```python
from build123d import *

# Parameters (mm, degrees)
F1_DEPTH  = 15.875
F2_W      = 4.318
F2_H      = 12.7
F3_DEPTH  = 9.175040233
F4_R      = 2.15899
F5_R      = 3.175
F6_DEPTH  = 3.81
F8_DEPTH  = 25.4
F10_DEPTH = 25.4
F11_R     = 3.175


# Not quite as in the source:
# - a fillet or chamfer is up to 0.001 mm smaller than in the source, because OpenCascade refuses the exact size


with BuildPart() as f1:
    # F0 (on Front) → F1 (new body)
    with BuildSketch(Plane.XZ):
        Polygon((9.2045814112, -87.6168819653), (3.0183370735, -43.5994663098), (0, -44.0236659215), (6.1862443377, -88.041081577), align=None)
    extrude(amount=F1_DEPTH)

    # F2 (on face) → F3 (cut, through all)
    with BuildSketch(Plane(origin=(-6.067283434, 0, -0.8527010782), x_dir=(0, -1, 0), z_dir=(-0.9902680687, 0, -0.139173101))):
        with Locations((7.9375, -54.072730631)):
            Rectangle(F2_W, F2_H)
        with Locations((7.9375, -76.297730631)):
            Rectangle(F2_W, F2_H)
    extrude(amount=-F3_DEPTH, mode=Mode.SUBTRACT)

    # F4 (radius 2.159 in the source; OpenCascade refuses exactly that, so slightly less here)
    f4_edges = [f1.edges().sort_by_distance(p)[0] for p in [
        (2.083606, -5.7785, -47.898898),
        (5.176728, -5.7785, -69.907605),
        (5.176728, -10.0965, -69.907605),
        (2.083606, -10.0965, -47.898898),
        (3.851104, -10.0965, -60.475302),
        (6.944226, -10.0965, -82.48401),
        (6.944226, -5.7785, -82.48401),
        (3.851104, -5.7785, -60.475302),
    ]]
    fillet(f4_edges, radius=F4_R)

    # F5 (on Front) → F6 (join)
    with BuildSketch(Plane.XZ):
        Polygon((9.2045814112, -87.6168819653), (3.0183370735, -43.5994663098), (-22.5109767612, -43.5994663098), (-22.5109767612, -25.4), (-73.3109767612, -25.4), (-73.3109767612, -87.6168819653), align=None)
        with Locations((-60.6109767612, -38.1)):
            Circle(F5_R, mode=Mode.SUBTRACT)
    extrude(amount=-F6_DEPTH)

    # F7 (on Front) → F8 (cut)
    with BuildSketch(Plane.XZ):
        Polygon((-73.3109767612, -38.1), (-60.6109767612, -25.4), (-73.3109767612, -25.4), align=None)
    extrude(amount=-F8_DEPTH, mode=Mode.SUBTRACT)

    # F9 (on Front) → F10 (cut)
    with BuildSketch(Plane.XZ):
        Polygon((-74.5969353161, -25.4), (-60.6109767612, -39.3859585549), (-52.9750182062, -31.75), (-22.5109767612, -31.75), (-22.5109767612, -25.4), align=None)
    extrude(amount=-F10_DEPTH, mode=Mode.SUBTRACT)

    # F11
    f11_edges = [f1.edges().sort_by_distance(p)[0] for p in [
        (-67.603956, 1.905, -32.392979),
    ]]
    fillet(f11_edges, radius=F11_R)


solid = f1.part
```
Geometry check sheet. Reference: the model listing, model coordinates, mm. A direction names the side the tool comes from. Give positions to 0.01 mm unless a question says otherwise; leave off trailing zeros. Order: outer loops, then holes, each group sorted by start corner. A loop starts at its lowest first (then second) coordinate and runs counter-clockwise, first axis right, second up. Notation, with made-up numbers: (-8, -18.75) - (24, -18.75) arc R24 ccw to (24, 16.25) - close; hole circle Ø6 at (51, 16). An arc over 180 degrees is marked (long way). Write item = value, one per line. Start each with the question number.
1) Section check B-B (x = -26). Enter the section's corners in (y, z), then the cut area to 3 significant figures.
2) Section check C-C (z = -62.5). Enter the section's corners in (x, y) (3 decimals), then the cut area to 3 significant figures.
3) Draft check along Z on faces 1 (the flat face through (-71.6, 1.88, -36.39)), 2 (the flat face through (3.05, -7.83, -65.72)), 3 (the cylindrical face through (5.288, -9.481, -70.548)). Enter one of: released by +Z, released by -Z, zero draft, split by the parting line, or undercut.
4) Section check D-D (x = -59). Enter the section's corners in (y, z).
5) Access from +Z, -Z, +X, -X, +Y, -Y to the whole of each face (thin tool, end or side, straight path). Record for faces 4 (the flat face through (1.53, -7.83, -43.81)), 5 (the cylindrical face through (3.787, -6.428, -59.863)), 6 (the flat face through (-55.43, 1.878, -34.205)), 7 (the flat face through (-22.511, 2, -38)).
6) Gauge pin test, flat ends, axial feed: pin 1 Ø3 at (y, z) = (-9.5, -81.5) entering from -X; pin 2 Ø5 at (y, z) = (-10.5, -81.5) entering from +X; pin 3 Ø12 at (x, z) = (-8, -38.5) entering from -Y. Record the tip position at first contact, or that the pin passes through.
7) Scan lines: L1, parallel to Y at x = -69, z = -71; L2, parallel to Z at x = -13, y = 2.75; L3, parallel to Z at x = -42.5, y = 2. Record each from-to range of solid material in increasing order.
8) Section check A-A (y = -7). Enter the section's corners in (x, z).
Geometry check:
q1.outline = (0, -87.62) - (3.81, -87.62) - (3.81, -31.75) - (0, -31.75) - close
q1.area = 213 mm2
q2.outline = (-73.311, 0) - (2.597, 0) - (2.597, -15.875) - (5.675, -15.875) - (5.675, 3.81) - (-73.311, 3.81) - close
q2.area = 350 mm2
q3.face_1 = released by +Z
q3.face_2 = released by -Z
q3.face_3 = undercut
q4.outline = (0, -87.62) - (3.81, -87.62) - (3.81, -40.84) - (0, -40.84) - close
q5.face_4 = +Z, -X, -Y
q5.face_5 = -X
q5.face_6 = +Z, +Y, -Y
q5.face_7 = +Z, +X, +Y, -Y
q6.pin_1 = 5.07
q6.pin_2 = 8.7
q6.pin_3 = 0
q7.L1 = 0 to 3.81
q7.L2 = -87.62 to -43.6
q7.L3 = -87.62 to -31.75
q8.outline = (0, -44.02) - (0.6, -48.32) - (3.62, -47.9) - (3.02, -43.6) - close; (2.31, -60.48) - (3.7, -70.33) - (6.72, -69.91) - (5.33, -60.05) - close; (5.41, -82.48) - (6.19, -88.04) - (9.2, -87.62) - (8.42, -82.06) - close
